from build123d import *

# Parameters (mm, degrees)
SKETCH_1_R               = 5
EXTRUDE_1_DEPTH          = 14
SKETCH_2_W               = 13.996795202
SKETCH_2_H               = 2
CUT_EXTRUDE_1_DEPTH      = 3
CUT_EXTRUDE_2_DEPTH      = 13
CUT_EXTRUDE_2_DEPTH_BACK = 13
SKETCH_3_R               = 3


with BuildPart() as part:
    # Sketch 1 → Extrude 1 (new body)
    with BuildSketch(Plane(origin=(0, 0, 0), x_dir=(1, 0, 0), z_dir=(0, 1, 0))):
        with Locations(Location((0, 0, 0), (0, 0, 270))):
            Circle(SKETCH_1_R)
    extrude(amount=EXTRUDE_1_DEPTH)

    # Sketch 2 → Cut-Extrude 1 (cut)
    with BuildSketch(Plane(origin=(0, 14, 0), x_dir=(1, 0, 0), z_dir=(0, 1, 0))):
        Rectangle(SKETCH_2_W, SKETCH_2_H)
    extrude(amount=-CUT_EXTRUDE_1_DEPTH, mode=Mode.SUBTRACT)

    # Sketch 3 → Cut-Extrude 2 (cut, two sides: drawn at the far end of the back side and taken through both)
    with BuildSketch(Plane(origin=(0, 0, 0), x_dir=(0, 0, -1), z_dir=(1, 0, 0)).offset(-CUT_EXTRUDE_2_DEPTH_BACK)):
        with Locations(Location((0, 5, 0), (0, 0, 180))):
            Circle(SKETCH_3_R)
    extrude(amount=CUT_EXTRUDE_2_DEPTH + CUT_EXTRUDE_2_DEPTH_BACK, mode=Mode.SUBTRACT)


solid = part.part
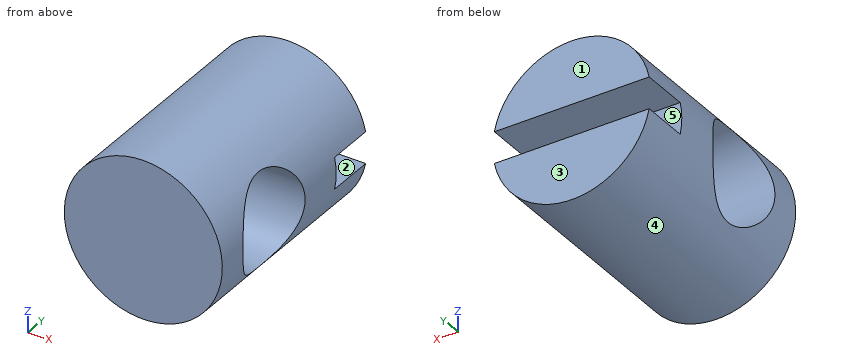
Input: part model. Units: mm. Frame: model coordinates. Face numbers are marked on the shaded views. A direction names the side the tool comes from. Round coordinates to 2 decimals unless told otherwise and drop trailing zeros. Write each loop counter-clockwise with the first axis right and the second up, starting at its lowest first coordinate (ties: lowest second). Pieces come first, ordered by that corner, then holes.
1) Reachability of the marked faces 1 and 2 from +Z, -Z, +X, -X, +Y, -Y: full face, straight path, thin tool, end or side. Return the list, or none.
2) Cut plane D-D (z = -1.5). Return the cut outline in (x, y).
3) Ray query, L1, parallel to Y at x = 2, z = 0; L2, parallel to Z at x = 3, y = 5; L3, parallel to Z at x = -0.5, y = 12. Return the intervals inside material, ascending.
4) Contact query for flat-ended pins moving along their axis: P1, Ø5, axis at y = 4.5, z = 1.5, coming from the -X side; P2, Ø2, axis at x = 0.5, y = 1.5, coming from the +Z side; P3, Ø1, axis at x = -2, z = 0, coming from the +Y side; P4, Ø2.5, axis at x = 2, y = 12.5, coming from the -Z side. Output: stop coordinate, or through.
5) Cut plane A-A (z = 0). Return the cut outline in (x, y).
6) Draft query along Z for the marked faces 3, 4 and 5. Return one class per face: pulls with the +Z half, pulls with the -Z half, needs draft (parallel to the pull), parting line crosses it, or undercut.
7) Cut plane B-B (x = 0). Return the cut outline in (y, z).
8) Cut plane C-C (y = 11.5). Return the cut outline in (x, z), then the cut area to 3 significant figures.
Geometry says:
1. face 1: +Z, -Z, +X, -X, +Y
1. face 2: +X, -X, +Y
2. outline: (-4.77, 0) - (4.77, 0) - (4.77, 2.4) - (-4.77, 2.4) - close; (-4.77, 7.6) - (4.77, 7.6) - (4.77, 14) - (-4.77, 14) - close
3. L1: y = 0 to 2, 8 to 11
3. L2: z = -4 to -3, 3 to 4
3. L3: z = -4.97 to -1, 1 to 4.97
4. P1: stops at x = -4.94
4. P2: stops at z = 5
4. P3: stops at y = 11
4. P4: stops at z = -4.94
5. outline: (-5, 0) - (5, 0) - (5, 2) - (-5, 2) - close; (-5, 8) - (5, 8) - (5, 11) - (-5, 11) - close
6. face 3: needs draft
6. face 4: parting line crosses it
6. face 5: undercut
7. outline: (0, -5) - (14, -5) - (14, -1) - (11, -1) - (11, 1) - (14, 1) - (14, 5) - (0, 5) - close; hole circle Ø6 at (5, 0)
8. outline: (-4.9, -1) arc R5 ccw to (4.9, -1) - close; (-4.9, 1) - (4.9, 1) arc R5 ccw to start
8. area: 58.7 mm2
